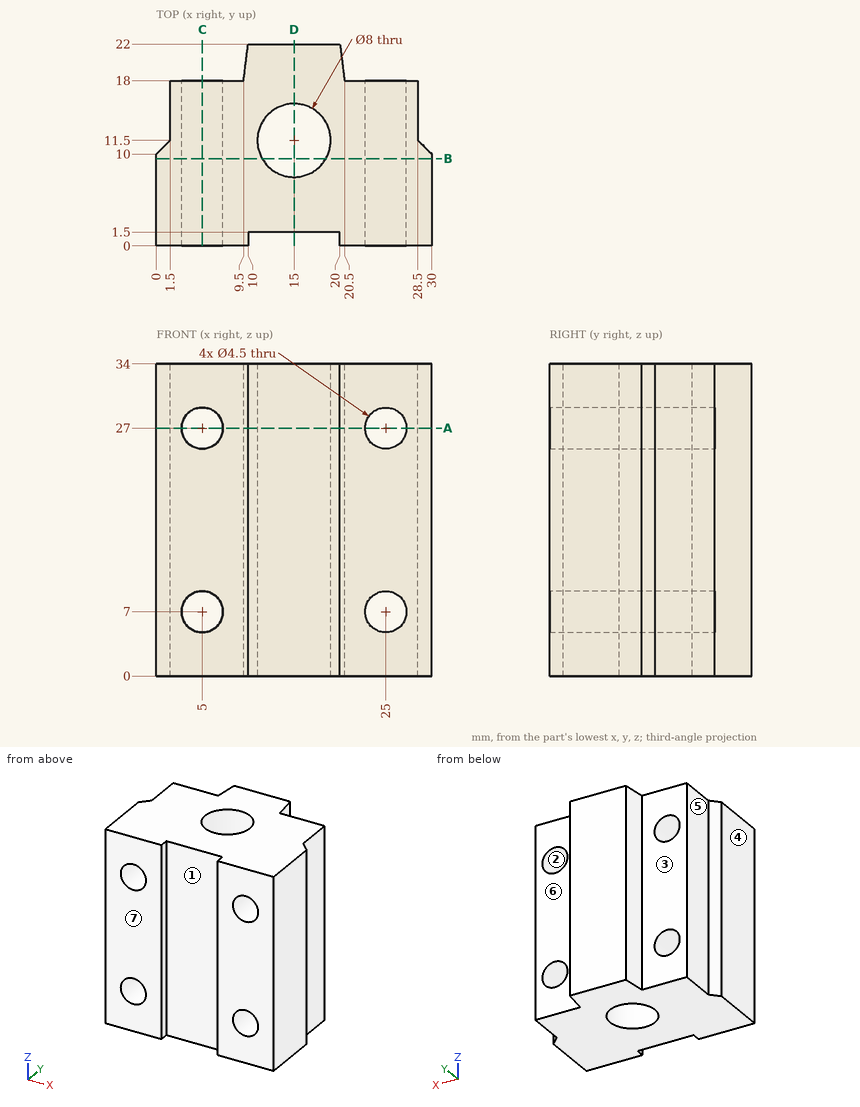
Could you check a few things on this drawing? It's one solid part, dimensions in mm from its lowest x, y, z. A direction names the side the tool comes from. Coordinates: 2 decimals unless noted, no trailing zeros. Order: outer loops, then holes, each group sorted by start corner. A loop starts at its lowest first (then second) coordinate and runs counter-clockwise, first axis right, second up.
1. If we section it at B-B (y = 9.5): Please give me the cut outline in (x, z).
2. For the marked faces 5, 6 and 7, which set-ups out of +Z, -Z, +X, -X, +Y, -Y let a thin tool reach every point of the face, with its end or its side?
3. If we section it at A-A (z = 27): Please give me the cut outline in (x, y), then the cut area to 3 significant figures.
4. I'm going to push flat-ended pins straight in: pin 1 (5 mm diameter, centred on x = 25, z = 27, fed in from +Y); pin 2 (7 mm diameter, centred on y = 14, z = 25.5, fed in from +X); pin 3 (5 mm diameter, centred on y = 16.5, z = 20.5, fed in from -X). Where does each tip first touch, or does it pass through?
5. If we section it at D-D (x = 15): Please give me the cut outline in (y, z), then the cut area to 3 significant figures.
6. Thinking about a two-plate mould opening in X: for the marked faces 1, 2, 3 and 4, which applies, +X half, -X half, draft (parallel to the pull), parting line (faces both ways), or undercut?
7. If we section it at C-C (x = 5): Please give me the cut outline in (y, z).
8. I need wall thicknesses on line 1 (Z direction, x = 5, y = 6.75); line 2 (X direction, y = 4, z = 27); line 3 (X direction, y = 1, z = 9.5). Which ranges of each line are inside material? Lowest first, please.
Entries:
1. outline: (0, 0) - (11.54, 0) - (11.54, 34) - (0, 34) - close; (18.46, 0) - (30, 0) - (30, 34) - (18.46, 34) - close; hole circle Ø4.5 at (5, 7); hole circle Ø4.5 at (5, 27); hole circle Ø4.5 at (25, 7); hole circle Ø4.5 at (25, 27)
2. face 5: +Z, -Z, -X, +Y
2. face 6: +Z, -Z, +X, +Y
2. face 7: +Z, -Z, +X, -X, -Y
3. outline: (0, 0) - (2.75, 0) - (2.75, 18) - (1.5, 18) - (1.5, 11.5) - (0, 10) - close; (7.25, 0) - (10, 0) - (10, 1.5) - (20, 1.5) - (20, 0) - (22.75, 0) - (22.75, 18) - (20.5, 18) - (20, 22) - (10, 22) - (9.5, 18) - (7.25, 18) - close; (27.25, 0) - (30, 0) - (30, 10) - (28.5, 11.5) - (28.5, 18) - (27.25, 18) - close; hole circle Ø8 at (15, 11.5)
3. area: 333 mm2
4. pin 1: stops at y = 18
4. pin 2: stops at x = 29.5
4. pin 3: stops at x = 1.5
5. outline: (1.5, 0) - (7.5, 0) - (7.5, 34) - (1.5, 34) - close; (15.5, 0) - (22, 0) - (22, 34) - (15.5, 34) - close
5. area: 425 mm2
6. face 1: undercut
6. face 2: undercut
6. face 3: draft
6. face 4: -X half
7. outline: (0, 0) - (18, 0) - (18, 4.75) - (0, 4.75) - close; (0, 9.25) - (18, 9.25) - (18, 24.75) - (0, 24.75) - close; (0, 29.25) - (18, 29.25) - (18, 34) - (0, 34) - close
8. line 1: z = 0 to 4.75, 9.25 to 24.75, 29.25 to 34
8. line 2: x = 0 to 2.75, 7.25 to 22.75, 27.25 to 30
8. line 3: x = 0 to 10, 20 to 30
